Geometry check sheet. Reference: the model listing, model coordinates, mm. Coordinates: 2 decimals unless noted, no trailing zeros. Order: outer loops, then holes, each group sorted by start corner. A loop starts at its lowest first (then second) coordinate and runs counter-clockwise, first axis right, second up.
```python
from build123d import *

# Parameters (mm, degrees)
SKETCH1_R           = 1.5
SKETCH1_W           = 3
SKETCH1_H           = 3
SKETCH1_H_2         = 10
BOSS_EXTRUDE1_DEPTH = 3


with BuildPart() as part:
    # Sketch1 → Boss-Extrude1 (new body)
    with BuildSketch(Plane(origin=(0, 0, 0), x_dir=(1, 0, 0), z_dir=(0, 1, 0))):
        with BuildLine():
            Line((256, 100), (256, 150))
            Line((256, 150), (253, 150))
            Line((253, 150), (253, 200))
            Line((253, 200), (256, 200))
            Line((256, 200), (256, 247))
            Line((256, 247), (203, 247))
            Line((203, 247), (203, 250))
            Line((203, 250), (153, 250))
            Line((153, 250), (153, 247))
            Line((153, 247), (103, 247))
            Line((103, 247), (103, 250))
            Line((103, 250), (53, 250))
            Line((53, 250), (53, 247))
            Line((53, 247), (-7, 247))
            ThreePointArc((-7, 247), (-9.121320344, 246.121320344), (-10, 244))
            Line((-10, 244), (-10, 240))
            ThreePointArc((-10, 240), (-9.121320344, 237.878679656), (-7, 237))
            Line((-7, 237), (0, 237))
            Line((0, 237), (0, 203))
            Line((0, 203), (3, 203))
            Line((3, 203), (3, 153))
            Line((3, 153), (0, 153))
            Line((0, 153), (0, 103))
            Line((0, 103), (3, 103))
            Line((3, 103), (3, 53))
            Line((3, 53), (0, 53))
            Line((0, 53), (0, 50))
            Line((0, 50), (-10.1, 50))
            ThreePointArc((-10.1, 50), (-13.635533906, 48.535533906), (-15.1, 45))
            Line((-15.1, 45), (-15.1, 43))
            Line((-15.1, 43), (-15.1, 21))
            ThreePointArc((-15.1, 21), (-14.221320344, 18.878679656), (-12.1, 18))
            Line((-12.1, 18), (-9.1, 18))
            ThreePointArc((-9.1, 18), (-6.978679656, 18.878679656), (-6.1, 21))
            Line((-6.1, 21), (-6.1, 40))
            Line((-6.1, 40), (0, 40))
            Line((0, 40), (0, 0))
            Line((0, 0), (0, -3))
            Line((0, -3), (3, -3))
            Line((3, -3), (3, 0))
            Line((3, 0), (53, 0))
            Line((53, 0), (53, -3))
            Line((53, -3), (103, -3))
            Line((103, -3), (103, 0))
            Line((103, 0), (153, 0))
            Line((153, 0), (153, -3))
            Line((153, -3), (203, -3))
            Line((203, -3), (203, 0))
            Line((203, 0), (256, 0))
            Line((256, 0), (256, 50))
            Line((256, 50), (253, 50))
            Line((253, 50), (253, 100))
            Line((253, 100), (256, 100))
        make_face()
        with Locations(Location((-5, 242, 0), (0, 0, 270))):
            Circle(SKETCH1_R, mode=Mode.SUBTRACT)
        with Locations((-10.6, 29.5)):
            Rectangle(SKETCH1_W, SKETCH1_H, mode=Mode.SUBTRACT)
        Polygon((184, 172), (234, 172), (234, 217), (22, 217), (22, 172), (72, 172), (72, 192), (81, 192), (81, 172), (175, 172), (175, 192), (184, 192), align=None, mode=Mode.SUBTRACT)
        with Locations((-10.6, 36.5)):
            Rectangle(SKETCH1_W, SKETCH1_H, mode=Mode.SUBTRACT)
        with Locations((4.5, 29.5)):
            Rectangle(SKETCH1_W, SKETCH1_H, mode=Mode.SUBTRACT)
        with Locations((4.5, 36.5)):
            Rectangle(SKETCH1_W, SKETCH1_H, mode=Mode.SUBTRACT)
        with Locations((76.5, 40)):
            Rectangle(SKETCH1_W, SKETCH1_H_2, mode=Mode.SUBTRACT)
        with Locations((179.5, 40)):
            Rectangle(SKETCH1_W, SKETCH1_H_2, mode=Mode.SUBTRACT)
        with Locations((76.5, 108.5)):
            Rectangle(SKETCH1_W, SKETCH1_H_2, mode=Mode.SUBTRACT)
        with Locations((179.5, 108.5)):
            Rectangle(SKETCH1_W, SKETCH1_H_2, mode=Mode.SUBTRACT)
        with Locations((76.5, 177)):
            Rectangle(SKETCH1_W, SKETCH1_H_2, mode=Mode.SUBTRACT)
        with Locations((179.5, 177)):
            Rectangle(SKETCH1_W, SKETCH1_H_2, mode=Mode.SUBTRACT)
        Polygon((22, 35), (72, 35), (72, 55), (81, 55), (81, 35), (175, 35), (175, 55), (184, 55), (184, 35), (234, 35), (234, 80), (22, 80), align=None, mode=Mode.SUBTRACT)
        Polygon((22, 103.5), (72, 103.5), (72, 123.5), (81, 123.5), (81, 103.5), (175, 103.5), (175, 123.5), (184, 123.5), (184, 103.5), (234, 103.5), (234, 148.5), (22, 148.5), align=None, mode=Mode.SUBTRACT)
    extrude(amount=BOSS_EXTRUDE1_DEPTH)


solid = part.part
```
Item 1: Sectioned sample at C-C (x = 17). Record the cut outline in (y, z).
Item 2: Sectioned sample at D-D (y = 1.95). Give the number of separate pieces and of enclosed holes in the cut face, and give its area (3 significant figures).
Item 3: Sectioned sample at A-A (z = -142.5). Record the cut outline in (x, y).
Item 4: Depth check by flat-ended pin: P1, Ø1.5, axis at x = 215, y = 0.5, coming from the -Z side; P2, Ø1.5, axis at y = 1.5, z = -199.5, coming from the -X side; P3, Ø1.5, axis at y = 1, z = 1, coming from the +X side. Enter the tip coordinate at first touch or a pass-through.
Item 5: Sectioned sample at B-B (x = 139). Record the cut outline in (y, z).
Item 6: Thickness scan on line 1 along Z through (x, y) = (51, 1.75); line 2 along X through (y, z) = (2.4, -28.5); line 3 along X through (y, z) = (1, -242). Record the ranges inside material, lowest first.
Geometry check:
1. outline: (0, -247) - (3, -247) - (3, 0) - (0, 0) - close
2. separate pieces: 1
2. enclosed holes: 14
2. area: 35,900 mm2
3. outline: (0, 0) - (22, 0) - (22, 3) - (0, 3) - close; (234, 0) - (256, 0) - (256, 3) - (234, 3) - close
4. P1: stops at z = -247
4. P2: stops at x = 3
4. P3: stops at x = 203
5. outline: (0, -247) - (3, -247) - (3, -217) - (0, -217) - close; (0, -172) - (3, -172) - (3, -148.5) - (0, -148.5) - close; (0, -103.5) - (3, -103.5) - (3, -80) - (0, -80) - close; (0, -35) - (3, -35) - (3, 0) - (0, 0) - close
6. line 1: z = -247 to -217, -172 to -148.5, -103.5 to -80, -35 to 0
6. line 2: x = -15.1 to -12.1, -9.1 to -6.1, 0 to 3, 6 to 256
6. line 3: x = -10 to -6.5, -3.5 to 256
